```python
from build123d import *

# Parameters (mm, degrees)
SKETCH_1_R      = 31.5
EXTRUDE_1_DEPTH = 10
FILLET_1_R      = 150
FILLET_3_R      = 15


with BuildPart() as part:
    # 草图1 → 凸台-拉伸1 (new body)
    with BuildSketch(Plane(origin=(0, 0, 0), x_dir=(1, 0, 0), z_dir=(0, 1, 0))):
        with Locations(Location((0, 0, 0), (0, 0, 270))):
            Circle(SKETCH_1_R)
    extrude(amount=EXTRUDE_1_DEPTH)

    # 草图3 → 旋转1 (revolve)
    with BuildSketch(Plane.XY, mode=Mode.PRIVATE) as revolve_1_sk:
        Polygon((0, 95), (15, 95), (15, 25), (31.5, 10), (0, 10), align=None)
    revolve(revolve_1_sk.sketch.rotate(Axis((0, 0, 0), (0, 1, 0)), 90), axis=Axis((0, 0, 0), (0, 1, 0)))

    # 圆角1
    # the kernel refuses this fillet: 150 mm, written as the material it adds along each edge
    with BuildSketch(Plane(origin=(0, 25, 0), x_dir=(0, 0, -1), z_dir=(1, 0, 0))) as fillet_1_piece_1:
        with BuildLine():
            CenterArc((165, 53.394078691), FILLET_1_R, 180, 27.126753117)
            Line((15, 53.394078691), (12, 53.394078691))
            Line((12, 53.394078691), (12, 0))
            Line((12, 0), (12.981981618, -2.21982022))
            ThreePointArc((12.981981618, -2.21982022), (21.231981618, -9.71982022), (28.83, -16.367881574))
            Line((28.83, -16.367881574), (31.5, -15))
        make_face()
    revolve(axis=Axis((0, 25, 0), (0, 1, 0)))

    # 圆角3
    fillet_3_edges = [part.edges().sort_by_distance(p)[0] for p in [
        (-31.5, 10, 0),
    ]]
    fillet(fillet_3_edges, radius=FILLET_3_R)


solid = part.part
```
Check sheet for the modelled part. Datum: model origin and axes. Units: mm. A direction names the side the tool comes from. Coordinates: 2 decimals unless noted, no trailing zeros. Write each loop counter-clockwise with the first axis right and the second up, starting at its lowest first coordinate (ties: lowest second). Pieces come first, ordered by that corner, then holes. Notation, with made-up numbers: M -32,9 L -2,9 A18 ccw -2,40 Z; hole C 48.25,-6 d11. An arc over 180 degrees is marked long. Use one line per item in the form item = value.
Item 1: Gauge pin test, flat ends, axial feed: pin 1 Ø3 at (x, y) = (-6, 30) entering from +Z; pin 2 Ø2 at (y, z) = (39.5, 18) entering from -X; pin 3 Ø4 at (y, z) = (49, -20) entering from -X; pin 4 Ø2 at (x, y) = (0.5, 35) entering from -Z. Record the tip position at first contact, or that the pin passes through.
Answer below:
pin_1 = 22.88
pin_2 = -10.86
pin_3 = through
pin_4 = -21.71
Item 2: Set-up check for faces 1 (the face through (-12.65, 86.58, -8.06)), 2 (the face through (9.462, 3.191, 30.045)): record each of +Z, -Z, +X, -X, +Y, -Y from which the full face is reachable in a straight line by a thin tool's end or side.
Answer below:
face_1 = +Y
face_2 = +Y, -Y
Item 3: Material ranges on L1, parallel to Z at x = 16, y = 43; L2, parallel to Z at x = 7.5, y = 54; L3, parallel to X at y = 62, z = 12.5, recorded low to high. Write a range as from..to.
Answer below:
L1 = -10.68..10.68
L2 = -15.25..15.25
L3 = -9.82..9.82
Item 4: Sectioned sample at B-B, the plane y = 62.5. Record the cut outline in (x, z), and give its area (3 significant figures).
Answer below:
outline = C 0,0 d31.69
area = 789 mm^2
Item 5: Sectioned sample at A-A, the plane y = 77. Record the cut outline in (x, z).
Answer below:
outline = C 0,0 d30.01
